from build123d import *

# Parameters (mm, degrees)
SCHIZZO1_R                   = 4
SCHIZZO1_R_2                 = 2
ESTRUSIONE_ESTRUSIONE1_DEPTH = 5


with BuildPart() as part:
    # Schizzo1 → Estrusione-Estrusione1 (new body)
    with BuildSketch(Plane.XY):
        with BuildLine():
            Line((14.409830056, 30.980762114), (-14.409830056, 30.980762114))
            ThreePointArc((-14.409830056, 30.980762114), (-26.495190528, 29.730762114), (-21.535042047, 18.639532931))
            Line((-21.535042047, 18.639532931), (-7.125211991, 2.341229183))
            ThreePointArc((-7.125211991, 2.341229183), (0, -7.5), (7.125211991, 2.341229183))
            Line((7.125211991, 2.341229183), (21.535042047, 18.639532931))
            ThreePointArc((21.535042047, 18.639532931), (26.495190528, 29.730762114), (14.409830056, 30.980762114))
        make_face()
        Circle(SCHIZZO1_R, mode=Mode.SUBTRACT)
        with Locations((20, 25.980762114)):
            Circle(SCHIZZO1_R_2, mode=Mode.SUBTRACT)
        with Locations((-20, 25.980762114)):
            Circle(SCHIZZO1_R_2, mode=Mode.SUBTRACT)
        Polygon((11, 20.980762114), (-11, 20.980762114), (0, 10), align=None, mode=Mode.SUBTRACT)
    extrude(amount=ESTRUSIONE_ESTRUSIONE1_DEPTH)


solid = part.part
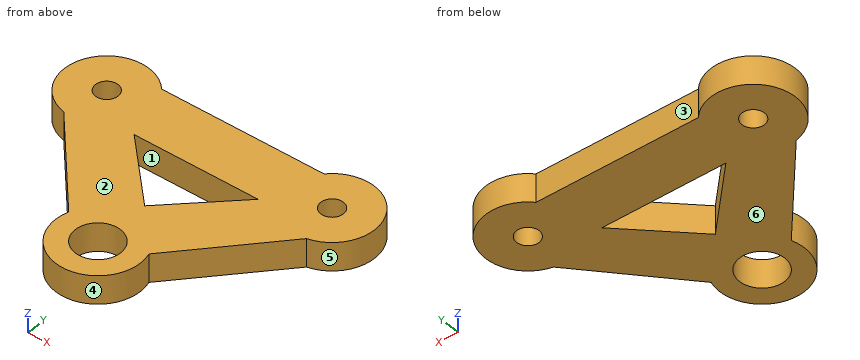
The listing builds one solid part. Answer for the finished solid, in the listing's coordinates (mm). Face numbers are marked on the shaded views. A direction names the side the tool comes from. Give positions to 0.01 mm unless a question says otherwise; leave off trailing zeros. Loops run counter-clockwise (first coordinate to the right, second up) from the corner with the lowest first, then second, coordinate; pieces in that order, holes last.
Item 1: Each of these flat-tipped pins is pushed along its axis until it touches: pin 1 Ø1.5 at (y, z) = (25, 1) entering from +X; pin 2 Ø3 at (x, z) = (18, 1.5) entering from -Y; pin 3 Ø2 at (y, z) = (28.5, 3) entering from -X. Where does it stop, or does it pass through?
Derived:
pin 1: stops at x = 27.5
pin 2: stops at y = 12.94
pin 3: stops at x = -27.34
Item 2: Determine the mould class of the marked faces 3, 4, 5 and 6 for opening direction Y: +Y half, -Y half, draft (parallel to the pull), parting line (faces both ways), or undercut.
Derived:
face 3: +Y half
face 4: undercut
face 5: parting line
face 6: draft
Item 3: A cutting plane is placed at A-A (y = 0). Give the vertices of the cut face in (x, z).
Derived:
outline: (-7.5, 0) - (-4, 0) - (-4, 5) - (-7.5, 5) - close; (4, 0) - (7.5, 0) - (7.5, 5) - (4, 5) - close
Item 4: A cutting plane is placed at D-D (x = 15.5). Give the vertices of the cut face in (y, z), then the cut area to 3 significant figures.
Derived:
outline: (11.81, 0) - (31.98, 0) - (31.98, 5) - (11.81, 5) - close
area: 101 mm2
Item 5: A cutting plane is placed at B-B (x = -20). Give the vertices of the cut face in (y, z), then the cut area to 3 significant figures.
Derived:
outline: (16.9, 0) - (23.98, 0) - (23.98, 5) - (16.9, 5) - close; (27.98, 0) - (33.48, 0) - (33.48, 5) - (27.98, 5) - close
area: 62.9 mm2
Item 6: A cutting plane is placed at C-C (z = 3.7). Give the vertices of the cut face in (x, y), then the cut area to 3 significant figures.
Derived:
outline: (-21.54, 18.64) - (-7.13, 2.34) arc R7.5 ccw (long way) to (7.13, 2.34) - (21.54, 18.64) arc R7.5 ccw (long way) to (14.41, 30.98) - (-14.41, 30.98) arc R7.5 ccw (long way) to start; hole circle Ø4 at (-20, 25.98); hole (-11, 20.98) - (0, 10) - (11, 20.98) - close; hole circle Ø8 at (0, 0); hole circle Ø4 at (20, 25.98)
area: 1,080 mm2
Item 7: A tool of negligible diameter and unlimited length cuts with its end or side. For the marked faces 1 and 2, from which of +Z, -Z, +X, -X, +Y, -Y can it reach the whole face along a straight path? Write none if from no direction.
Derived:
face 1: +Z, -Z
face 2: +Z, +X, -X, +Y, -Y
Item 8: Find the intervals of material crossed by line 1 along X through (y, z) = (25, 1.9); line 2 along Y through (x, z) = (-20, 1.5); line 3 along X through (y, z) = (32.5, 2.15), in increasing order.
Derived:
line 1: x = -27.44 to -21.74, -18.26 to 18.26, 21.74 to 27.44
line 2: y = 16.9 to 23.98, 27.98 to 33.48
line 3: x = -23.71 to -16.29, 16.29 to 23.71
